Check sheet for the drawn part. Datum: minimum x, y, z corner. Units: mm. A direction names the side the tool comes from. Round coordinates to 2 decimals unless told otherwise and drop trailing zeros. Order: outer loops, then holes, each group sorted by start corner. A loop starts at its lowest first (then second) coordinate and runs counter-clockwise, first axis right, second up.
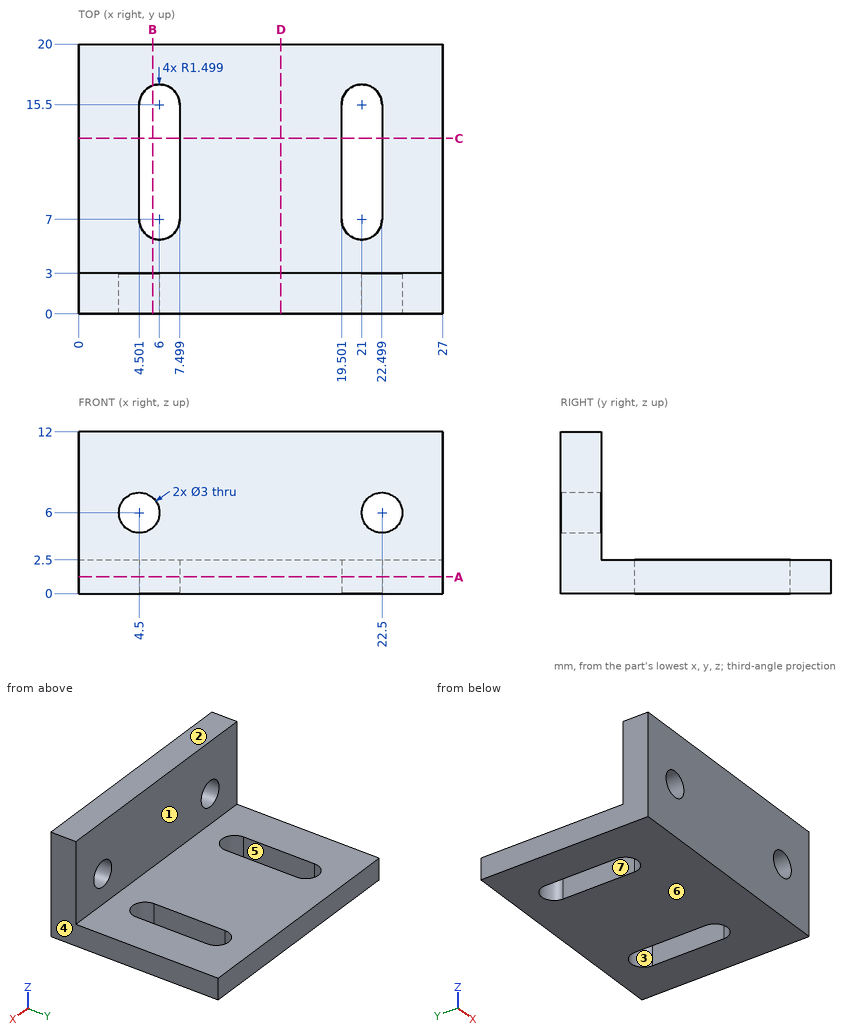
1) Gauge pin test, flat ends, axial feed: pin 1 (5 mm diameter, centred on x = 12.5, y = 15, fed in from +Z); pin 2 (1.2 mm diameter, centred on y = 13.5, z = 2, fed in from -X); pin 3 (1.8 mm diameter, centred on x = 22.5, z = 6, fed in from +Y). Record the tip position at first contact, or that the pin passes through.
2) Draft check along X on the marked faces 4, 5, 6 and 7. Enter one of: pulls with the +X half, pulls with the -X half, needs draft (parallel to the pull), parting line crosses it, or undercut.
3) Sectioned sample at C-C on y = 13. Record the cut outline in (x, z).
4) Sectioned sample at A-A on z = 1.25. Record the cut outline in (x, y), and give its area (3 significant figures).
5) Set-up check for the marked faces 1, 2 and 3: record each of +Z, -Z, +X, -X, +Y, -Y from which the full face is reachable in a straight line by a thin tool's end or side.
6) Sectioned sample at B-B on x = 5.5. Record the cut outline in (y, z).
7) Sectioned sample at D-D on x = 15. Record the cut outline in (y, z).
8) Scan lines: line 1 (X direction, y = 1.7, z = 6); line 2 (X direction, y = 2.5, z = 7.25); line 3 (Z direction, x = 4.5, y = 0.95). Record each from-to range of solid material in increasing order.
Values found:
1. pin 1: stops at z = 2.5
1. pin 2: stops at x = 0
1. pin 3: passes through
2. face 4: pulls with the +X half
2. face 5: undercut
2. face 6: needs draft
2. face 7: undercut
3. outline: (0, 0) - (4.5, 0) - (4.5, 2.5) - (0, 2.5) - close; (7.5, 0) - (19.5, 0) - (19.5, 2.5) - (7.5, 2.5) - close; (22.5, 0) - (27, 0) - (27, 2.5) - (22.5, 2.5) - close
4. outline: (0, 0) - (27, 0) - (27, 20) - (0, 20) - close; hole (4.5, 7) arc R1.5 ccw to (7.5, 7) - (7.5, 15.5) arc R1.5 ccw to (4.5, 15.5) - close; hole (19.5, 7) arc R1.5 ccw to (22.5, 7) - (22.5, 15.5) arc R1.5 ccw to (19.5, 15.5) - close
4. area: 475 mm2
5. face 1: +Z, +X, -X, +Y
5. face 2: +Z, +X, -X, +Y, -Y
5. face 3: +Z, -Z
6. outline: (0, 0) - (5.59, 0) - (5.59, 2.5) - (3, 2.5) - (3, 4.88) - (0, 4.88) - close; (0, 7.12) - (3, 7.12) - (3, 12) - (0, 12) - close; (16.91, 0) - (20, 0) - (20, 2.5) - (16.91, 2.5) - close
7. outline: (0, 0) - (20, 0) - (20, 2.5) - (3, 2.5) - (3, 12) - (0, 12) - close
8. line 1: x = 0 to 3, 6 to 21, 24 to 27
8. line 2: x = 0 to 3.67, 5.33 to 21.67, 23.33 to 27
8. line 3: z = 0 to 4.5, 7.5 to 12
